Autodesk Inventor part; units mm, degrees
ref_plane "Płaszczyzna konstrukcyjna1" through (0, 0, -30) normal (0, 0, -1) x (-1, 0, 0)
ref_plane "Płaszczyzna konstrukcyjna2" through (0, 0, -20) normal (0, 0, -1) x (-1, 0, 0)
ref_plane "Płaszczyzna konstrukcyjna3" through (0, 0, 0) normal (0, 0, -1) x (-1, 0, 0)
sketch "Szkic1" plane through (0, 0, 0) normal (0, 0, 1) x (1, 0, 0)
  line L0 (-55, -55) -> (55, -55)
  line L1 (55, -55) -> (55, 55)
  line L2 (55, 55) -> (-55, 55)
  line L3 (-55, 55) -> (-55, -55)
  line L4 (-55, -55) -> (55, 55) construction
  line L5 (-55, 55) -> (-55, 40) construction
  line L6 (-55, 40) -> (-50, 40)
  line L7 (-50, 40) -> (50, 40)
  line L8 (50, 40) -> (50, -2)
  line L9 (50, -2) -> (-50, -2)
  line L10 (-50, -2) -> (-50, 40)
  line L11 (0, -2) -> (0, -27) construction
  circle A0 centre (0, -27) radius 2
  line L12 (0, -27) -> (27.5, -27) construction
  line L13 (27.5, -27) -> (-27.5, -27) construction
  circle A1 centre (-27.5, -27) radius 10.5
  circle A2 centre (27.5, -27) radius 9.5
  line L14 (0, -27) -> (0, -47) construction
  line L15 (0, -47) -> (0, -57) construction
  line L16 (0, -47) -> (-18, -47) construction
  line L17 (-18, -47) -> (-36, -47) construction
  line L18 (0, -47) -> (18, -47) construction
  line L19 (18, -47) -> (36, -47) construction
  circle A3 centre (-36, -47) radius 2.5
  circle A4 centre (-18, -47) radius 2.5
  circle A5 centre (0, -47) radius 2.5
  circle A6 centre (18, -47) radius 2.5
  circle A7 centre (36, -47) radius 2.5
  line L20 (-57.5, -57.5) -> (57.5, -57.5)
  line L21 (57.5, -57.5) -> (57.5, 57.5)
  line L22 (57.5, 57.5) -> (-57.5, 57.5)
  line L23 (-57.5, 57.5) -> (-57.5, -57.5)
  line L24 (-57.5, -57.5) -> (57.5, 57.5) construction
  line L25 (57.5, -57.5) -> (-57.5, 57.5) construction
  point P0 (0, 0)
  point P1 (-55, -37)
  point P2 (55, -37)
  dimension "d0" = 110
  dimension "d1" = 110
  dimension "d2" = 15
  dimension "d3" = 100
  dimension "d4" = 42
  dimension "d5" = 25
  dimension "d6" = 4
  dimension "d7" = 27.5
  dimension "d8" = 55
  dimension "d10" = 19
  dimension "d11" = 20
  dimension "d12" = 10
  dimension "d13" = 18
  dimension "d14" = 18
  dimension "d15" = 18
  dimension "d16" = 18
  dimension "d17" = 5
  dimension "d18" = 5
  dimension "d19" = 5
  dimension "d20" = 5
  dimension "d21" = 5
  dimension "d51" = 115
  dimension "d52" = 115
extrude "Wyciągnięcie proste1" add sketch "Szkic1" along normal blind 1.5 contours L3 L2 L1 L0 | L23 L22 L21 L20
ref_plane "Płaszczyzna konstrukcyjna1" through (0, 0, -30) normal (0, 0, -1) x (-1, 0, 0)
ref_plane "Płaszczyzna konstrukcyjna2" through (0, 0, -20) normal (0, 0, -1) x (-1, 0, 0)
ref_plane "Płaszczyzna konstrukcyjna3" through (0, 0, 0) normal (0, 0, -1) x (-1, 0, 0)
ref_plane "Płaszczyzna konstrukcyjna4" through (75, -75, -30) normal (0, 0, -1) x (-1, 0, 0)
chamfer "Faza1" [suppressed]
sketch "Szkic9" plane through (0, 0, 0) normal (0, 0, -1) x (-1, 0, 0)
  line L0 (-57.5, -57.5) -> (57.5, -57.5)
  line L1 (57.5, -57.5) -> (57.5, 57.5)
  line L2 (57.5, 57.5) -> (-57.5, 57.5)
  line L3 (-57.5, 57.5) -> (-57.5, -57.5)
  line L4 (-57.5, -57.5) -> (57.5, 57.5) construction
  line L5 (57.5, -57.5) -> (-57.5, 57.5) construction
  point P0 (0, 0)
sketch "Szkic10" plane through (0, 0, 0) normal (0, 0, -1) x (-1, 0, 0)
  line L0 (-55, -55) -> (55, -55)
  line L1 (55, -55) -> (55, 55)
  line L2 (55, 55) -> (-55, 55)
  line L3 (-55, 55) -> (-55, -55)
  line L4 (-55, -55) -> (55, 55) construction
  line L5 (55, -55) -> (-55, 55) construction
  point P0 (0, 0)
  dimension "d67" = 110
  dimension "d68" = 110
ref_plane "Płaszczyzna konstrukcyjna5" through (45.0845, 55, -30) normal (0, 0, -1) x (-1, 0, 0)
sketch "Szkic14" plane through (45.0845, 55, -30) normal (0, 0, -1) x (-1, 0, 0)
  line L0 (-19.9155, -130) -> (110.0845, -130)
  line L1 (110.0845, -130) -> (110.0845, 20)
  line L2 (110.0845, 20) -> (-19.9155, 20)
  line L3 (-19.9155, 20) -> (-19.9155, -130)
  line L4 (-19.9155, -130) -> (110.0845, 20) construction
  line L5 (110.0845, -130) -> (-19.9155, 20) construction
  point P0 (45.0845, -55)
  dimension "d93" = 130
  dimension "d94" = 150
sketch "Szkic15" plane through (45.0845, 55, -30) normal (0, 0, -1) x (-1, 0, 0)
  line L0 (107.5845, -127.5) -> (-17.4155, -127.5)
  line L1 (-17.4155, -127.5) -> (-17.4155, 17.5)
  line L2 (-17.4155, 17.5) -> (107.5845, 17.5)
  line L3 (107.5845, 17.5) -> (107.5845, -127.5)
  line L4 (107.5845, -127.5) -> (-17.4155, 17.5) construction
  line L5 (-17.4155, -127.5) -> (107.5845, 17.5) construction
  point P0 (45.0845, -55)
  dimension "d95" = 125
  dimension "d96" = 145
loft "Wyciągnięcie złożone5" add profiles "Szkic9", "Szkic14"
loft "Wyciągnięcie złożone6" cut profiles "Szkic15", "Szkic10"
sketch "Szkic8" plane through (0, 0, -20) normal (0, 0, -1) x (-1, 0, 0)
  line L0 (-52.5, -52.5) -> (52.5, 52.5) construction
  line L1 (-55, 55) -> (-62.5, 72.5)
  line L2 (52.5, 52.5) -> (52.5, 47.5)
  line L3 (52.5, 47.5) -> (38.6222, 60.8006)
  line L4 (57.5113, 42.6971) -> (52.5, 47.5)
  line L5 (-52.5, 52.5) -> (-47.5006, 52.5806)
  line L6 (-47.5006, 52.5806) -> (-33.6043, 66.9631)
  line L7 (-47.5006, 52.5806) -> (-60.6627, 38.958)
  line L8 (-60.6627, 38.958) -> (-60.1271, 66.9631)
  line L9 (-60.1271, 66.9631) -> (-33.6043, 66.9631)
  line L10 (-52.5, -52.5) -> (-42.5, -52.5)
  line L11 (-42.5, -52.5) -> (-60.3532, -35.2504)
  line L12 (45.4959, -47.1074) -> (40.6649, -52.1074)
  line L13 (45.4959, -47.1074) -> (60.2173, -31.8709)
  line L14 (-60.3532, -35.2504) -> (-60.3532, -67.4907)
  line L15 (-55, -55) -> (-62.5, -72.5)
  line L16 (-42.5, -52.5) -> (-34.5509, -60.4491)
  line L17 (-42.5, -52.5) -> (-31.2582, -52.5) construction
  line L18 (-60.3532, -67.4907) -> (-27.5093, -67.4907)
  line L19 (-27.5093, -67.4907) -> (-35.5667, -59.4333)
  line L20 (57.5113, 42.6971) -> (38.6222, 60.8006)
  line L21 (38.6222, 60.8006) -> (32.1923, 66.9631)
  line L22 (32.1923, 66.9631) -> (60.2173, 66.9631)
  line L23 (60.2173, 66.9631) -> (60.4778, 39.854)
  line L24 (60.4778, 39.854) -> (57.5113, 42.6971)
  line L25 (40.6649, -52.1074) -> (27.9311, -65.2867)
  line L26 (27.9311, -65.2867) -> (61.4401, -66.3113)
  line L27 (60.2173, -31.8709) -> (61.4401, -66.3113)
  point P0 (0, 0)
  dimension "d83" = 5
  dimension "d84" = 5
  dimension "d85" = 10
  dimension "d87" = 45
extrude "Wyciągnięcie proste3" add sketch "Szkic8" against normal up to next
properties part number "gora_obodowy_plaska"
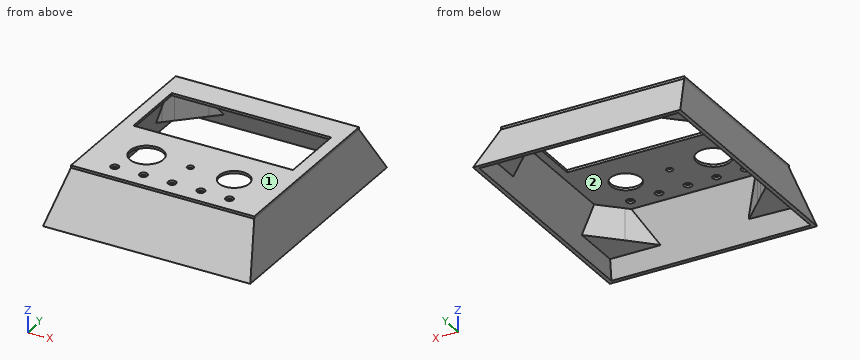
CAD build for the part. Positions are in the model's coordinates, mm. Face numbers are marked on the shaded views. Round coordinates to 2 decimals unless told otherwise and drop trailing zeros. Return JSON: item names as keys, results as strings. Group by question number.
Q1. Flat gauge pins, fed straight in: pin 1 Ø12 at (x, y) = (-26.5, -47) entering from -Z; pin 2 Ø9.5 at (x, y) = (-44, -56) entering from -Z; pin 3 Ø4 at (y, z) = (30.5, -19) entering from +X. Where does each tip first touch, or does it go through?
Q2. Drill centre lines: line 1 along Y through (x, z) = (-27.5, 0.45); line 2 along Y through (x, z) = (-18, 1); line 3 along Y through (x, z) = (35, -16.5) (3 decimals). Where is each one in solid material? Low to high. Write a range as [from, to].
Q3. Band-saw the part on A-A on y = -20.5. Give the number of separate pieces and of enclosed holes in the cut face, plus the area to 3 significant figures.
Q4. Two-plate mould, pull along Y, no slides. Class the marked faces 1 and 2: +Y half, -Y half, draft (parallel to the pull), parting line (faces both ways), or undercut.
Solutions:
{
 "1": {"pin 1": "stops at z = 0", "pin 2": "stops at z = -20", "pin 3": "stops at x = 62.75"},
 "2": {"line 1": "y = [-57.5, -37.5], [-16.5, -2], [40, 57.5]", "line 2": "y = [-57.5, -49.5], [-44.5, -31.47], [-22.53, -2], [40, 57.5]", "line 3": "y = [-67.125, -60], [64.625, 67.125]"},
 "3": {"separate pieces": "3", "enclosed holes": "0", "area": "277 mm^2"},
 "4": {"face 1": "draft", "face 2": "undercut"}
}
